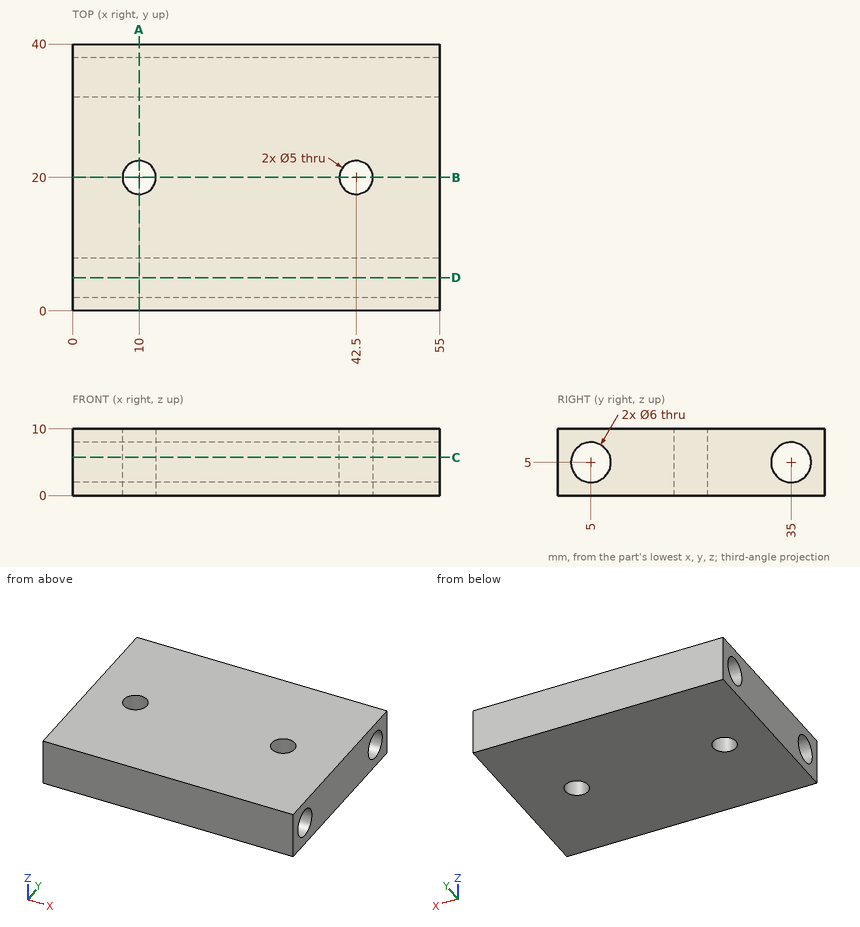
Study the drawing (mm; zero at the part's minimum x, y, z) and answer. Coordinates: 2 decimals unless noted, no trailing zeros. Loops run counter-clockwise (first coordinate to the right, second up) from the corner with the lowest first, then second, coordinate; pieces in that order, holes last. Notation, with made-up numbers: M -1.75,-16 L 15.25,-16 A18 ccw 15.25,6 Z; hole C 11.25,24.25 d10. An arc over 180 degrees is marked long. Answer in a Markdown table with one row per item. Add a question column.
1. Find section B-B, the plane y = 20. Write down the section's boundary in (x, z), then the cut area to 3 significant figures.
2. Find section C-C, the plane z = 5.75. Write down the section's boundary in (x, y), then the cut area to 3 significant figures.
3. Find section A-A, the plane x = 10. Write down the section's boundary in (y, z), then the cut area to 3 significant figures.
4. Consider L1, parallel to Y at x = 35.5, z = 5.25; L2, parallel to Z at x = 19.5, y = 5; L3, parallel to Y at x = 42.5, z = 2.25. Determine where each line is inside the solid, lowest interval first.
5. Find section D-D, the plane y = 5. Write down the section's boundary in (x, z).
Reported:
| question | item | result |
|---|---|---|
| 1 | outline | M 0,0 L 7.5,0 L 7.5,10 L 0,10 Z; M 12.5,0 L 40,0 L 40,10 L 12.5,10 Z; M 45,0 L 55,0 L 55,10 L 45,10 Z |
| 1 | area | 450 mm^2 |
| 2 | outline | M 0,0 L 55,0 L 55,2.1 L 0,2.1 Z; M 0,7.9 L 55,7.9 L 55,32.1 L 0,32.1 Z; M 0,37.9 L 55,37.9 L 55,40 L 0,40 Z; hole C 10,20 d5; hole C 42.5,20 d5 |
| 2 | area | 1,520 mm^2 |
| 3 | outline | M 0,0 L 17.5,0 L 17.5,10 L 0,10 Z; M 22.5,0 L 40,0 L 40,10 L 22.5,10 Z; hole C 5,5 d6; hole C 35,5 d6 |
| 3 | area | 293 mm^2 |
| 4 | L1 | y = 0 to 2.01, 7.99 to 32.01, 37.99 to 40 |
| 4 | L2 | z = 0 to 2, 8 to 10 |
| 4 | L3 | y = 0 to 3.8, 6.2 to 17.5, 22.5 to 33.8, 36.2 to 40 |
| 5 | outline | M 0,0 L 55,0 L 55,2 L 0,2 Z; M 0,8 L 55,8 L 55,10 L 0,10 Z |
